Check sheet for the drawn part. Datum: minimum x, y, z corner. Units: mm. Give positions to 0.01 mm unless a question says otherwise; leave off trailing zeros. Write each loop counter-clockwise with the first axis right and the second up, starting at its lowest first coordinate (ties: lowest second). Pieces come first, ordered by that corner, then holes. Notation, with made-up numbers: (76.5, 31.5) - (89.5, 31.5) arc R36 cw to (89.5, 67.5) - close; hole circle Ø1 at (63, 77). An arc over 180 degrees is marked (long way). Use a Markdown table: item, result.
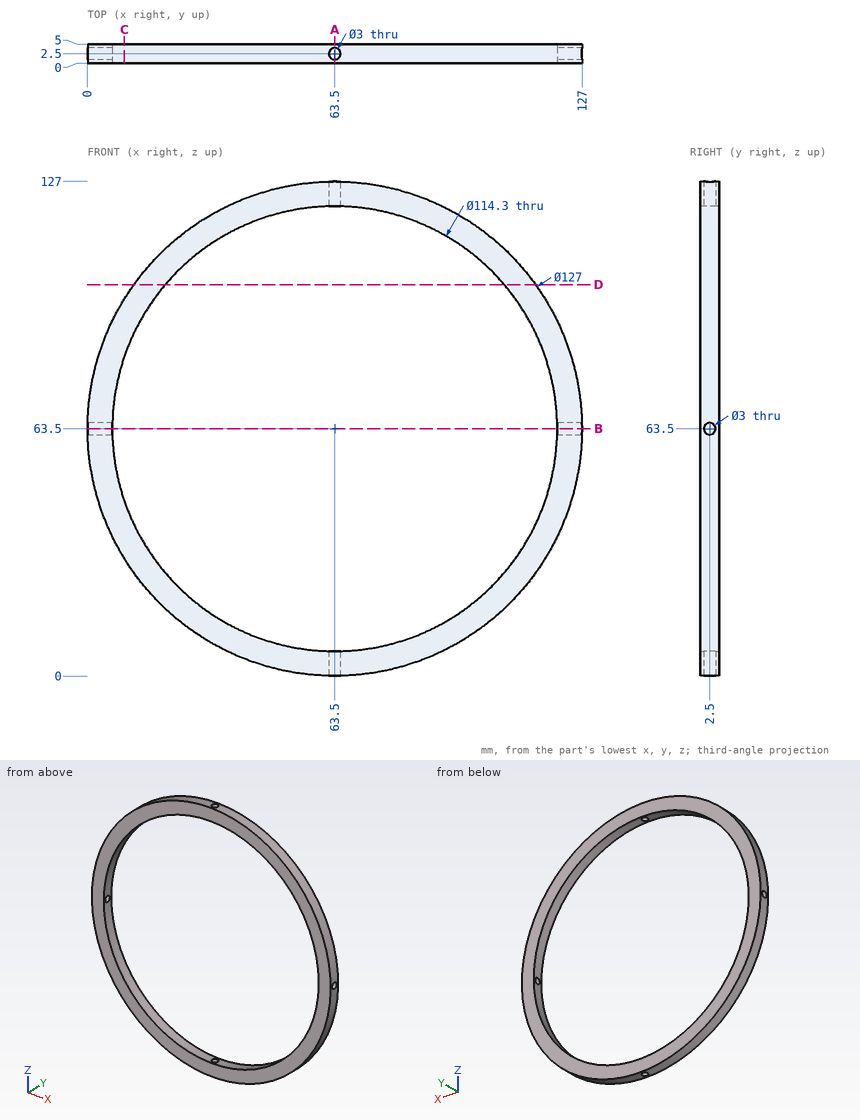
1) Section check A-A on x = 63.5. Record the boundary of the cut face in (y, z).
Working result:
| item | result |
|---|---|
| outline | (0, 0) - (1, 0) - (1, 6.35) - (0, 6.35) - close; (0, 120.65) - (1, 120.65) - (1, 127) - (0, 127) - close; (4, 0) - (5, 0) - (5, 6.35) - (4, 6.35) - close; (4, 120.65) - (5, 120.65) - (5, 127) - (4, 127) - close |
2) Section check C-C on x = 9.5. Record the boundary of the cut face in (y, z), then the cut area to 3 significant figures.
Working result:
| item | result |
|---|---|
| outline | (0, 30.09) - (5, 30.09) - (5, 44.79) - (0, 44.79) - close; (0, 82.21) - (5, 82.21) - (5, 96.91) - (0, 96.91) - close |
| area | 147 mm² |
3) Section check D-D on z = 100.5. Record the boundary of the cut face in (x, y), then the cut area to 3 significant figures.
Working result:
| item | result |
|---|---|
| outline | (11.89, 0) - (19.94, 0) - (19.94, 5) - (11.89, 5) - close; (107.06, 0) - (115.11, 0) - (115.11, 5) - (107.06, 5) - close |
| area | 80.5 mm² |
4) Depth check by flat-ended pin: P1, Ø1, axis at y = 2.5, z = 87.5, coming from the +X side; P2, Ø1, axis at x = 75, y = 2.5, coming from the -Z side; P3, Ø2, axis at y = 4, z = 76, coming from the -X side. Enter the tip coordinate at first touch or a pass-through.
Working result:
| item | result |
|---|---|
| P1 | stops at x = 122.49 |
| P2 | stops at z = 0.96 |
| P3 | stops at x = 1.05 |
5) Section check B-B on z = 63.5. Record the boundary of the cut face in (x, y), then the cut area to 3 significant figures.
Working result:
| item | result |
|---|---|
| outline | (0, 0) - (6.35, 0) - (6.35, 1) - (0, 1) - close; (0, 4) - (6.35, 4) - (6.35, 5) - (0, 5) - close; (120.65, 0) - (127, 0) - (127, 1) - (120.65, 1) - close; (120.65, 4) - (127, 4) - (127, 5) - (120.65, 5) - close |
| area | 25.4 mm² |
6) Material ranges on L1, parallel to Y at x = 2, z = 63.5; L2, parallel to X at y = 4.3, z = 63; L3, parallel to X at y = 3.1, z = 95, recorded low to high. Write a range as from..to.
Working result:
| item | result |
|---|---|
| L1 | y = 0..1, 4..5 |
| L2 | x = 0..6.35, 120.65..127 |
| L3 | x = 8.36..15.81, 111.19..118.64 |
